from build123d import *

# Parameters (mm, degrees)
F0_W     = 47
F0_H     = 27
F1_DEPTH = 17.5
F0_W_2   = 50
F0_H_2   = 30
F2_DEPTH = 3.5
F3_W     = 16.5
F3_H     = 24.5
F4_DEPTH = 19.5
F5_SIZE  = 4.5
F6_SIZE  = 5
F7_R     = 1.5


with BuildPart() as f1:
    # F0 (on Top) → F1 (new body)
    with BuildSketch(Plane.XY):
        Rectangle(F0_W, F0_H)
    extrude(amount=-F1_DEPTH)

    # F0 (on Top) → F2 (join)
    with BuildSketch(Plane.XY):
        Rectangle(F0_W_2, F0_H_2)
        Rectangle(F0_W, F0_H, mode=Mode.SUBTRACT)
        Rectangle(F0_W, F0_H)
    extrude(amount=F2_DEPTH)

    # F3 (on face) → F4 (cut)
    with BuildSketch(Plane.XY.offset(3.5)):
        with Locations((13.75, 0)):
            Rectangle(F3_W, F3_H)
    extrude(amount=-F4_DEPTH, mode=Mode.SUBTRACT)

    # F5
    f5_edges = [f1.edges().sort_by_distance(p)[0] for p in [
        (22, 12.25, -6.25),
        (22, -12.25, -6.25),
    ]]
    chamfer(f5_edges, length=F5_SIZE)

    # F6
    f6_edges = [f1.edges().sort_by_distance(p)[0] for p in [
        (23.5, 13.5, -8.75),
        (23.5, -13.5, -8.75),
    ]]
    chamfer(f6_edges, length=F6_SIZE)

    # F7
    f7_edges = [f1.edges().sort_by_distance(p)[0] for p in [
        (-25, 0, 3.5),
        (0, 15, 3.5),
        (25, 0, 3.5),
        (0, -15, 3.5),
        (25, -15, 1.75),
        (25, 15, 1.75),
        (-25, -15, 1.75),
        (-25, 15, 1.75),
    ]]
    fillet(f7_edges, radius=F7_R)


solid = f1.part
Here's how the part is built. I have some questions about the finished solid (model axes, mm). A direction names the side the tool comes from. Coordinates: 2 decimals unless noted, no trailing zeros. Order: outer loops, then holes, each group sorted by start corner. A loop starts at its lowest first (then second) coordinate and runs counter-clockwise, first axis right, second up. Notation, with made-up numbers: M 3.5,8.5 L 14.5,8.5 A10 ccw 14.5,12.5 Z; hole C 67,-10.75 d8. An arc over 180 degrees is marked long. Answer as CSV lines item,"result". Start each with the question number.
1. For pin 1 (5 mm diameter, centred on x = 0.5, z = -8, fed in from -Y); pin 2 (12 mm diameter, centred on x = -19, z = -14.5, fed in from +Y); pin 3 (5 mm diameter, centred on y = 10, z = -10.5, fed in from -X), each with a flat end and sliding along its axis, tell me the tip position at first contact or that it passes through.
2. I want a section at C-C, the plane y = -9.25. Write out the boundary of the cut face in (x, z).
3. I want a section at D-D, the plane x = 21.5. Write out the boundary of the cut face in (y, z), and give its area (3 significant figures).
4. I want a section at B-B, the plane x = -8. Write out the boundary of the cut face in (y, z), and give its area (3 significant figures).
5. I need wall thicknesses on line 1 (X direction, y = -3.25, z = -11.75); line 2 (Y direction, x = 17.5, z = 0.25); line 3 (X direction, y = -6, z = 1). Which ranges of each line are inside material? Lowest first, please. Write a range as [from, to].
6. I want a section at A-A, the plane z = -6.5. Write out the boundary of the cut face in (x, y), and give its area (3 significant figures).
7. We'd pull the mould along Y, two halves only. Please class faces 4 (the flat face through (23.5, 0, -9)), 5 (the flat face through (19.78, -9.97, -6.11)), 6 (the flat face through (21, 11, -9)): released by +Y, released by -Y, zero draft, split by the parting line, or undercut.
8. On a 3-axis mill with a long thin cutter (end or side, diameter ignored), from which of +Z, -Z, +X, -X, +Y, -Y can I reach the whole of each face in a straight line? I mean faces 1 (the flat face through (0, 0, -17.5)), 2 (the flat face through (-23.5, 0, -9)), 3 (the flat face through (5.5, 0, -6)). Say none if no direction works.
Recorded:
1,pin 1,"stops at y = -13.5"
1,pin 2,"stops at y = 13.5"
1,pin 3,"stops at x = -23.5"
2,outline,"M -25,0 L -23.5,0 L -23.5,-17.5 L 22.75,-17.5 L 22.75,0 L 25,0 L 25,2 A1.5 ccw 23.5,3.5 L 20.5,3.5 L 20.5,-16 L 5.5,-16 L 5.5,3.5 L -23.5,3.5 A1.5 ccw -25,2 Z"
3,outline,"M -15,0 L -10.5,0 L -10.5,-17.5 L 10.5,-17.5 L 10.5,0 L 15,0 L 15,2 A1.5 ccw 13.5,3.5 L 8.25,3.5 L 8.25,-16 L -8.25,-16 L -8.25,3.5 L -13.5,3.5 A1.5 ccw -15,2 Z"
3,area,"150 mm2"
4,outline,"M -15,0 L -13.5,0 L -13.5,-17.5 L 13.5,-17.5 L 13.5,0 L 15,0 L 15,2 A1.5 ccw 13.5,3.5 L -13.5,3.5 A1.5 ccw -15,2 Z"
4,area,"577 mm2"
5,line 1,"x = [-23.5, 5.5], [22, 23.5]"
5,line 2,"y = [-15, -12.25], [12.25, 15]"
5,line 3,"x = [-25, 5.5], [22, 25]"
6,outline,"M -23.5,-13.5 L 18.5,-13.5 L 23.5,-8.5 L 23.5,8.5 L 18.5,13.5 L -23.5,13.5 Z; hole M 5.5,-12.25 L 17.5,-12.25 L 22,-7.75 L 22,7.75 L 17.5,12.25 L 5.5,12.25 Z"
6,area,"860 mm2"
7,face 4,"zero draft"
7,face 5,"undercut"
7,face 6,"released by +Y"
8,face 1,"-Z, +X, -X, +Y, -Y"
8,face 2,"-Z, -X, +Y, -Y"
8,face 3,"+Z"
